```python
from build123d import *

# Parameters (mm, degrees)
SKETCH1_R                  = 36
BOSS_EXTRUDE1_DEPTH        = 38
FILLET1_R                  = 10
SKETCH2_R                  = 1.99
CUT_EXTRUDE1_DEPTH         = 39
M20X1_5_TAPPED_HOLE1_D     = 18.5
M20X1_5_TAPPED_HOLE1_DEPTH = 30
M20X1_5_TAPPED_HOLE1_TIP   = 5.557960726
M30X1_5_TAPPED_HOLE1_D     = 28.5
M30X1_5_TAPPED_HOLE1_DEPTH = 30
M30X1_5_TAPPED_HOLE1_TIP   = 8.562263821


with BuildPart() as part:
    # Sketch1 → Boss-Extrude1 (new body)
    with BuildSketch(Plane(origin=(0, 0, 0), x_dir=(1, 0, 0), z_dir=(0, 1, 0))):
        with BuildLine():
            Line((150, 0), (-150, 0))
            Line((-150, 0), (-150, 186))
            ThreePointArc((-150, 186), (-182.334192428, 252.209125332), (-110.238209296, 237))
            Line((-110.238209296, 237), (110.238209296, 237))
            ThreePointArc((110.238209296, 237), (182.334192428, 252.209125332), (150, 186))
            Line((150, 186), (150, 0))
        make_face()
        with Locations((-150, 227)):
            Circle(SKETCH1_R, mode=Mode.SUBTRACT)
        with Locations((150, 227)):
            Circle(SKETCH1_R, mode=Mode.SUBTRACT)
    extrude(amount=BOSS_EXTRUDE1_DEPTH)

    # Fillet1
    fillet1_edges = [part.edges().sort_by_distance(p)[0] for p in [
        (-150, 19, -186),
        (-110.238209296, 19, -237),
        (110.238209296, 19, -237),
        (150, 19, -186),
    ]]
    fillet(fillet1_edges, radius=FILLET1_R)

    # Sketch2 → Cut-Extrude1 (cut, through all)
    with BuildSketch(Plane(origin=(0, 38, 0), x_dir=(1, 0, 0), z_dir=(0, 1, 0))):
        with Locations((-10.25, 33.3)):
            Circle(SKETCH2_R)
        with Locations((10.25, 145.68)):
            Circle(SKETCH2_R)
    extrude(amount=-CUT_EXTRUDE1_DEPTH, mode=Mode.SUBTRACT)

    # M20x1.5 Tapped Hole1
    with Locations(Plane(origin=(0, 0, 0), x_dir=(-1, 0, 0), z_dir=(0, -1, 0))):
        with Locations((42.25, 145.68), (-42.25, 145.68), (42.25, 33.3), (-42.25, 33.3)):
            Hole(M20X1_5_TAPPED_HOLE1_D / 2, depth=M20X1_5_TAPPED_HOLE1_DEPTH)
            with Locations((0, 0, -(M20X1_5_TAPPED_HOLE1_DEPTH + M20X1_5_TAPPED_HOLE1_TIP / 2))):  # 118° drill point
                Cone(0, M20X1_5_TAPPED_HOLE1_D / 2, M20X1_5_TAPPED_HOLE1_TIP, mode=Mode.SUBTRACT)

    # M30x1.5 Tapped Hole1
    with Locations(Plane(origin=(0, 38, 0), x_dir=(1, 0, 0), z_dir=(0, 1, 0))):
        with Locations((0, 89.74)):
            Hole(M30X1_5_TAPPED_HOLE1_D / 2, depth=M30X1_5_TAPPED_HOLE1_DEPTH)
            with Locations((0, 0, -(M30X1_5_TAPPED_HOLE1_DEPTH + M30X1_5_TAPPED_HOLE1_TIP / 2))):  # 118° drill point
                Cone(0, M30X1_5_TAPPED_HOLE1_D / 2, M30X1_5_TAPPED_HOLE1_TIP, mode=Mode.SUBTRACT)


solid = part.part
```
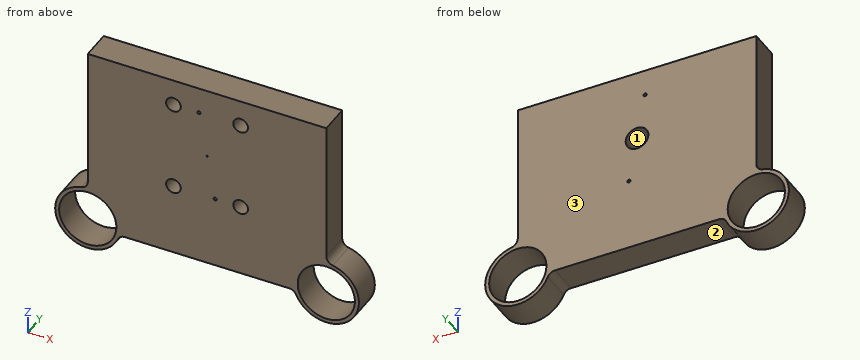
Model file for the job. Use its own axes, mm. Face numbers are marked on the shaded views. A direction names the side the tool comes from. Coordinates: 2 decimals unless noted, no trailing zeros. Order: outer loops, then holes, each group sorted by start corner. A loop starts at its lowest first (then second) coordinate and runs counter-clockwise, first axis right, second up. Notation, with made-up numbers: (19, 88) - (72, 88) arc R17 cw to (72, 93) - close; hole circle Ø8 at (69, 24). An arc over 180 degrees is marked (long way). Return JSON: item names as keys, results as strings. Group by question number.
1) Saw through at D-D, the plane z = -68.5. Write the cut outline in (x, y).
2) Saw through at B-B, the plane x = 125. Write the cut outline in (y, z), plus the area to 3 significant figures.
3) Probe line 1 (X direction, y = 21, z = -33.3); line 2 (Z direction, x = 42.25, y = 23); line 3 (Z direction, x = -10, y = 30). List the from-to ranges inside material, lowest first. Write a range as from..to.
4) Flat gauge pins, fed straight in: P1, Ø19, axis at y = 21, z = -89, coming from the +X side; P2, Ø19, axis at x = -14.5, y = 19, coming from the -Z side; P3, Ø10, axis at y = 32.5, z = -217, coming from the +X side; P4, Ø3.5, axis at x = -10.25, z = -33.3, coming from the -Y side. Where does each tip first touch, or does it go through?
5) Saw through at A-A, the plane z = -227. Write the cut outline in (x, y), plus the area to 3 significant figures.
6) Tool access for the marked faces 1, 2 and 3: list every direction of +Z, -Z, +X, -X, +Y, -Y with a clear straight run to the whole face (end or side of a thin tool).
7) Saw through at C-C, the plane x = 82. Write the cut outline in (y, z).
Values found:
{
 "1": {"outline": "(-150, 0) - (150, 0) - (150, 38) - (-150, 38) - close"},
 "2": {"outline": "(0, -259.5) - (38, -259.5) - (38, -252.9) - (0, -252.9) - close; (0, -201.1) - (38, -201.1) - (38, 0) - (0, 0) - close", "area": "7,890 mm²"},
 "3": {"line 1": "x = -150..-51.5, -33..-12.24, -8.26..33, 51.5..150", "line 2": "z = -237..-154.93, -136.43..-42.55, -24.05..0", "line 3": "z = -237..-99.89, -79.59..-35.27, -31.33..0"},
 "4": {"P1": "stops at x = 150", "P2": "stops at z = -237", "P3": "stops at x = 190.69", "P4": "passes through"},
 "5": {"outline": "(-191, 0) - (-186, 0) - (-186, 38) - (-191, 38) - close; (-114, 0) - (114, 0) - (114, 38) - (-114, 38) - close; (186, 0) - (191, 0) - (191, 38) - (186, 38) - close", "area": "9,040 mm²"},
 "6": {"face 1": "+Y", "face 2": "-Z, +Y, -Y", "face 3": "+Z, -Z, +X, -X, +Y"},
 "7": {"outline": "(0, -237) - (38, -237) - (38, 0) - (0, 0) - close"}
}
